Verification items for this drawing (mm, ordinates from the low corner). Give positions to 0.01 mm unless a question says otherwise; leave off trailing zeros. Order: outer loops, then holes, each group sorted by start corner. A loop starts at its lowest first (then second) coordinate and runs counter-clockwise, first axis right, second up. Notation, with made-up numbers: M -9.75,21.5 L 16.25,21.5 A23 cw 16.25,50.5 Z; hole C 14.25,59 d3. An arc over 180 degrees is marked long. One line per question, with ' | ' between items. Start each with the question number.
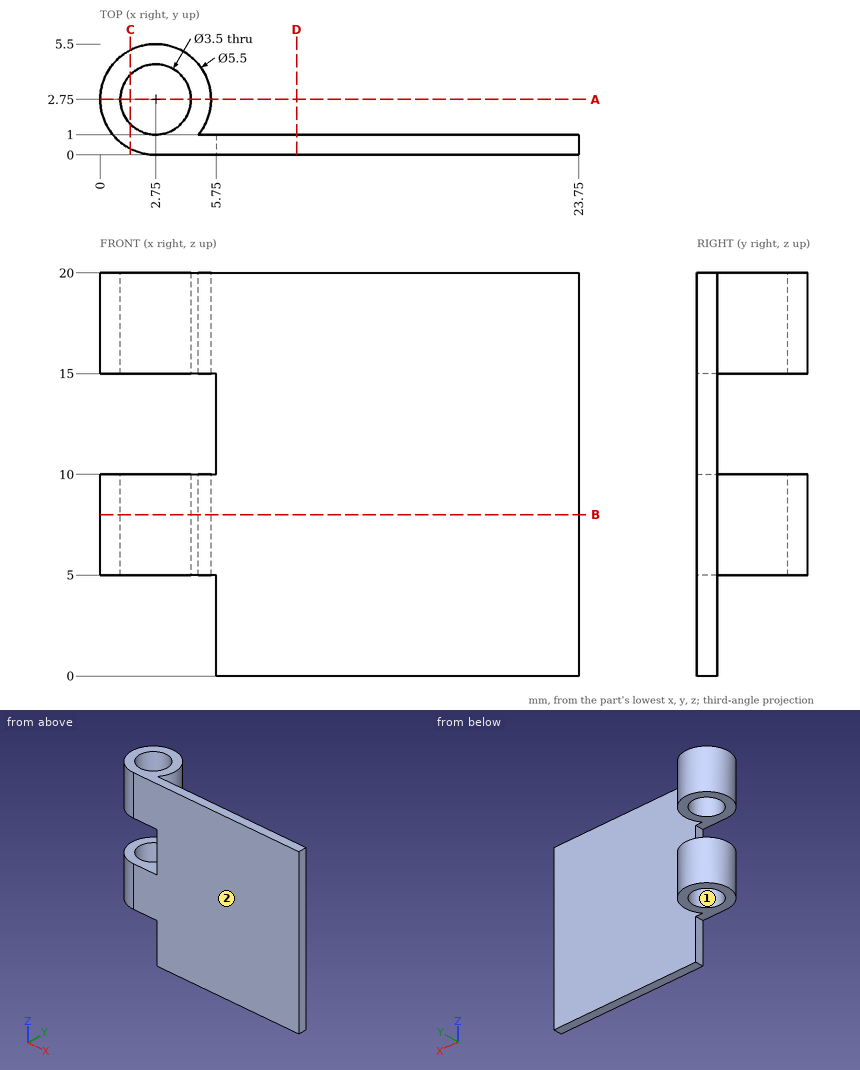
Item 1: Material ranges on line 1 along X through (y, z) = (2.75, 6.2); line 2 along Y through (x, z) = (12.75, 5.25), recorded low to high.
Item 2: Cross-section at B-B, the plane z = 8. Record the cut outline in (x, y), plus the area to 3 significant figures.
Item 3: Depth check by flat-ended pin: pin 1 (2 mm diameter, centred on x = 2.75, y = 2.75, fed in from +Z); pin 2 (6 mm diameter, centred on x = 20, z = 16, fed in from -Y); pin 3 (6 mm diameter, centred on x = 17.5, z = 16, fed in from +Y); pin 4 (3 mm diameter, centred on y = 1, z = 4.5, fed in from -X). Enter the tip coordinate at first touch or a pass-through.
Item 4: Mould release check, pull along X, two halves, no side actions. Record for the marked faces 1 and 2: released by +X, released by -X, zero draft, split by the parting line, or undercut.
Item 5: Cross-section at C-C, the plane x = 1.5. Record the cut outline in (y, z).
Item 6: Cross-section at D-D, the plane x = 9.75. Record the cut outline in (y, z), plus the area to 3 significant figures.
Item 7: Cross-section at A-A, the plane y = 2.75. Record the cut outline in (x, z), plus the area to 3 significant figures.
Outcome:
1) line 1: x = 0 to 1, 4.5 to 5.5 | line 2: y = 0 to 1
2) outline: M 2.75,0 L 23.75,0 L 23.75,1 L 4.87,1 A2.75 ccw long Z; hole C 2.75,2.75 d3.5 | area: 33.7 mm²
3) pin 1: passes through | pin 2: stops at y = 0 | pin 3: stops at y = 1 | pin 4: stops at x = 0.02
4) face 1: undercut | face 2: zero draft
5) outline: M 0.3,5 L 1.53,5 L 1.53,10 L 0.3,10 Z; M 0.3,15 L 1.53,15 L 1.53,20 L 0.3,20 Z; M 3.97,5 L 5.2,5 L 5.2,10 L 3.97,10 Z; M 3.97,15 L 5.2,15 L 5.2,20 L 3.97,20 Z
6) outline: M 0,0 L 1,0 L 1,20 L 0,20 Z | area: 20.0 mm²
7) outline: M 0,5 L 1,5 L 1,10 L 0,10 Z; M 0,15 L 1,15 L 1,20 L 0,20 Z; M 4.5,5 L 5.5,5 L 5.5,10 L 4.5,10 Z; M 4.5,15 L 5.5,15 L 5.5,20 L 4.5,20 Z | area: 20.0 mm²
